Here's the drawing with two shaded views (mm, measured from the low corner). I have some questions. Round coordinates to 2 decimals unless told otherwise and drop trailing zeros. Loops run counter-clockwise (first coordinate to the right, second up) from the corner with the lowest first, then second, coordinate; pieces in that order, holes last. Notation, with made-up numbers: (-21, 7) -> (21, 7) arc R13 ccw to (21, 18) -> close; hole circle Ø9 at (24, -33). An arc over 180 degrees is marked (long way). Write each question's results on one line, items separated by ' | '. Start each with the question number.
1) If I drill on probe 1 along X at (y, z) = (1.85, 19.25) (1 decimal); probe 2 along Z at (x, y) = (2.5, 2.1); probe 3 along X at (y, z) = (1.95, 22) (1 decimal), over which ranges is the centre line in solid material (lowest first)?
2) Imagine slicing it at B-B, the plane x = 22.5. List the corners of the cut face in (y, z) for me, plus the area to 3 significant figures.
3) Imagine slicing it at C-C, the plane y = 2.15. List the corners of the cut face in (x, z) for me (1 decimal), plus the area to 3 significant figures.
4) For P1, Ø1, axis at y = 2, z = 23.5, coming from the -X side, with a flat end and sliding along its axis, tell me the tip position at first contact or that it passes through.
5) We'd pull the mould along X, two halves only. Please class the marked faces 1 and 2: pulls with the +X half, pulls with the -X half, needs draft (parallel to the pull), parting line crosses it, or undercut.
6) Imagine slicing it at A-A, the plane z = 19.25. List the corners of the cut face in (x, y) for me (1 decimal).
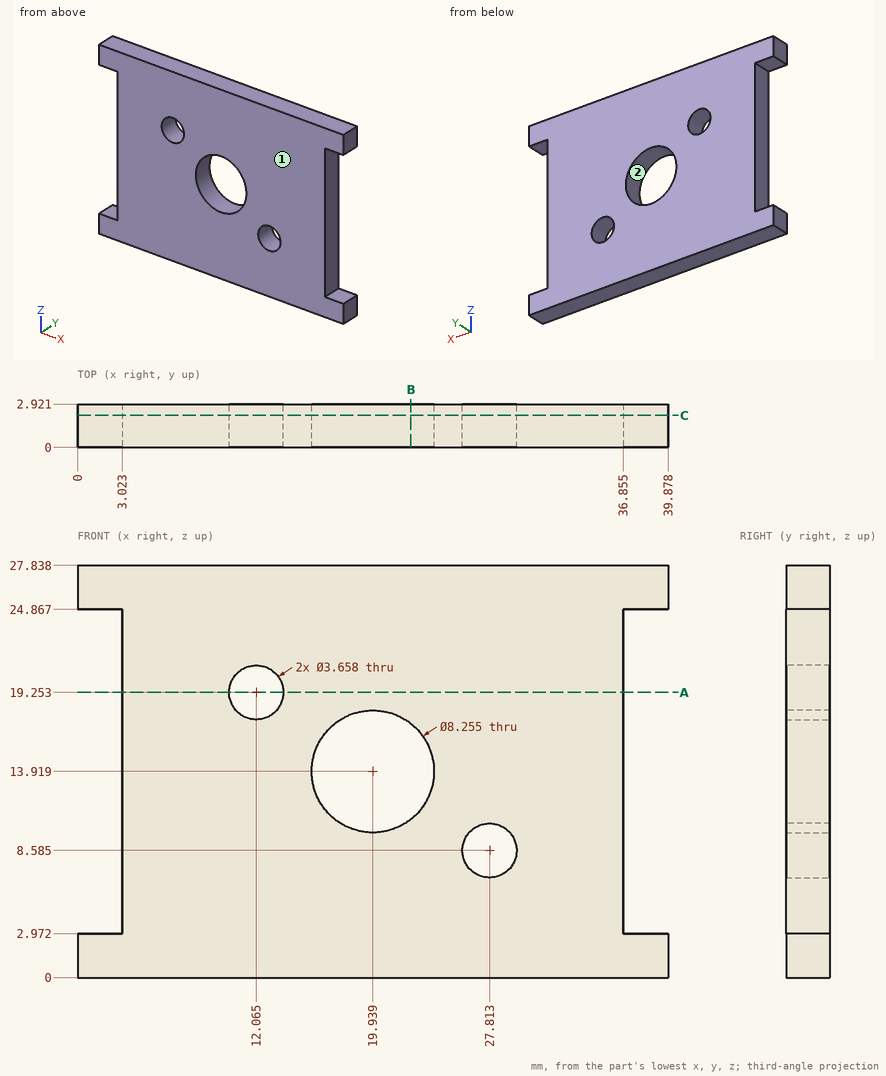
Checked values:
1) probe 1: 3 to 10.2, 13.9 to 36.9 | probe 2: 0 to 2.97, 24.87 to 27.84 | probe 3: 3 to 36.9
2) outline: (0, 0) -> (2.92, 0) -> (2.92, 10.68) -> (0, 10.68) -> close; (0, 17.16) -> (2.92, 17.16) -> (2.92, 27.84) -> (0, 27.84) -> close | area: 62.4 mm^2
3) outline: (0, 0) -> (39.9, 0) -> (39.9, 3) -> (36.9, 3) -> (36.9, 24.9) -> (39.9, 24.9) -> (39.9, 27.8) -> (0, 27.8) -> (0, 24.9) -> (3, 24.9) -> (3, 3) -> (0, 3) -> close; hole circle Ø3.7 at (12.1, 19.3); hole circle Ø8.3 at (19.9, 13.9); hole circle Ø3.7 at (27.8, 8.6) | area: 903 mm^2
4) P1: x = 3.02
5) face 1: needs draft | face 2: undercut
6) outline: (3, 0) -> (10.2, 0) -> (10.2, 2.9) -> (3, 2.9) -> close; (13.9, 0) -> (36.9, 0) -> (36.9, 2.9) -> (13.9, 2.9) -> close
